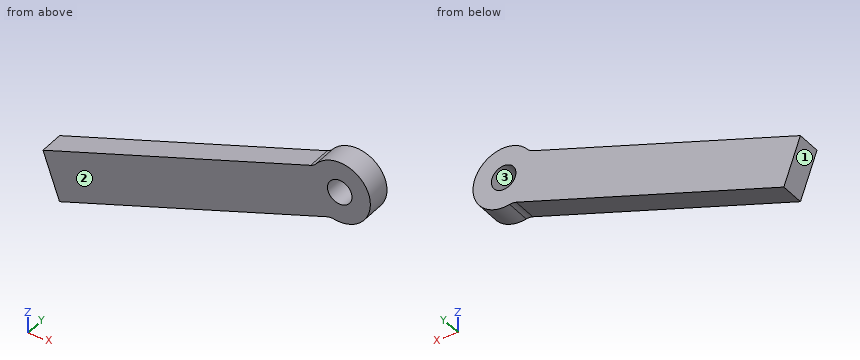
```python
from build123d import *

# Parameters (mm, degrees)
SKETCH1_R           = 1
BOSS_EXTRUDE1_DEPTH = 2


with BuildPart() as part:
    # Sketch1 → Boss-Extrude1 (new body)
    with BuildSketch(Plane(origin=(0, 0, 0), x_dir=(1, 0, 0), z_dir=(0, 1, 0))):
        with BuildLine():
            Line((-1.022874436, 2.490728385), (-22.861764958, 10.312114381))
            Line((-22.861764958, 10.312114381), (-24.21044114, 6.546337894))
            Line((-24.21044114, 6.546337894), (-2.371550618, -1.275048103))
            ThreePointArc((-2.371550618, -1.275048103), (-2.132203917, -1.399406187), (-1.93479976, -1.583208732))
            ThreePointArc((-1.93479976, -1.583208732), (2.353610305, -0.842922614), (-0.489789565, 2.451551791))
            ThreePointArc((-0.489789565, 2.451551791), (-0.758998088, 2.434862033), (-1.022874436, 2.490728385))
        make_face()
        Circle(SKETCH1_R, mode=Mode.SUBTRACT)
    extrude(amount=BOSS_EXTRUDE1_DEPTH)


solid = part.part
```
Design review of the part built by this model. Coordinates are the model's own, in mm. Face numbers are marked on the shaded views. Coordinates: 2 decimals unless noted, no trailing zeros. Loops run counter-clockwise (first coordinate to the right, second up) from the corner with the lowest first, then second, coordinate; pieces in that order, holes last.
Q1. We need section C-C on z = 0. State the section outline as (x, y) points.
Reported:
outline: (-5.93, 0) - (-1, 0) - (-1, 2) - (-5.93, 2) - close; (1, 0) - (2.5, 0) - (2.5, 2) - (1, 2) - close
Q2. To check wall thickness, follow line 1 (Z direction, x = 0, y = 0.4); line 2 (Z direction, x = -15, y = 1.75); line 3 (Z direction, x = -15.75, y = 0.75). State the ranges of each line that lie inside material, in increasing order.
Reported:
line 1: z = -2.5 to -1, 1 to 2.5
line 2: z = -7.5 to -3.25
line 3: z = -7.77 to -3.52
Q3. We need section B-B on y = 0.4. State the section outline as (x, z) points.
Reported:
outline: (-24.21, -6.55) - (-22.86, -10.31) - (-1.02, -2.49) arc R1 cw to (-0.49, -2.45) arc R2.5 ccw (long way) to (-1.93, 1.58) arc R1 cw to (-2.37, 1.28) - close; hole circle Ø2 at (0, 0)
Q4. We need section D-D on z = -8.5. State the section outline as (x, y) points, and give its area (3 significant figures).
Reported:
outline: (-23.51, 0) - (-17.8, 0) - (-17.8, 2) - (-23.51, 2) - close
area: 11.4 mm2
Q5. The part is to be moulded in two halves that separate along Z. For the marked faces 1, 2 and 3, say which applies: +Z half, -Z half, draft (parallel to the pull), parting line (faces both ways), or undercut.
Reported:
face 1: -Z half
face 2: draft
face 3: undercut
Q6. We need section A-A on x = 0. State the section outline as (y, z) points.
Reported:
outline: (0, -2.5) - (2, -2.5) - (2, -1) - (0, -1) - close; (0, 1) - (2, 1) - (2, 2.5) - (0, 2.5) - close
